Model file for the job. Use its own axes, mm. A direction names the side the tool comes from. Round coordinates to 2 decimals unless told otherwise and drop trailing zeros. Order: outer loops, then holes, each group sorted by start corner. A loop starts at its lowest first (then second) coordinate and runs counter-clockwise, first axis right, second up. Notation, with made-up numbers: (29, 45.25) - (58, 45.25) arc R26 cw to (58, 61.25) - close; hole circle Ø4 at (24, 35). An arc over 180 degrees is marked (long way). Put each result on its own line as item: value. Start each with the question number.
Item 1: Mould opens along Z. For faces 4 (the face through (2, 13, 2.075)), 5 (the face through (-1.5, 5.42, 0.07)), 6 (the face through (3, 15, -2.095)) say: pulls with the +Z half, pulls with the -Z half, needs draft (parallel to the pull), parting line crosses it, or undercut.
Item 2: Pin check, flat tips, straight feed: pin 1 Ø0.9 at (x, z) = (0, 0.5) entering from -Y; pin 2 Ø2 at (x, y) = (-2.5, 4) entering from -Z; pin 3 Ø3 at (x, y) = (2.5, 13.5) entering from +Z (3 decimals). Stop position of each tip, or through.
Item 3: Saw through at B-B on z = 0. List the corners of the cut face in (x, y).
Item 4: Saw through at D-D on z = -1.85. List the corners of the cut face in (x, y), plus the area to 3 significant figures.
Item 5: Saw through at C-C on y = 3.25. List the corners of the cut face in (x, z), plus the area to 3 significant figures.
Item 6: Which spindle directions (+Z, -Z, +X, -X, +Y, -Y) get a long thin tool onto all of the face, cutting with end or side? Do faces 1 (the face through (1.2, 12, -2.075)), 2 (the face through (-0.029, 10.166, 2.409)), 3 (the face through (-2.947, 5.916, -0.13)). Say none if no direction does.
Item 7: Probe probe 1 along Z at (x, y) = (0, 7.5); probe 2 along Z at (x, y) = (2.5, 16.75) (3 decimals); probe 3 along X at (y, z) = (13.25, -1.8). List the from-to ranges inside material, lowest first.
Item 8: Saw through at A-A on x = 0. List the corners of the cut face in (y, z) (3 decimals), plus the area to 3 significant figures.
```python
from build123d import *

# Parameters (mm, degrees)
SKETCH1_R               = 2.95
BOSS_EXTRUDE1_DEPTH     = 12
SKETCH5_R               = 1.5
CUT_EXTRUDE3_DEPTH      = 11
CUT_EXTRUDE4_DEPTH      = 5.5
CUT_EXTRUDE4_DEPTH_BACK = 5.5
SKETCH12_R              = 3.400000058
SKETCH12_R_2            = 2.501374622
BOSS_EXTRUDE5_DEPTH     = 0.02


with BuildPart() as part:
    # Sketch1 → Boss-Extrude1 (new body)
    with BuildSketch(Plane(origin=(0, 0, 0), x_dir=(1, 0, 0), z_dir=(0, 1, 0))):
        Circle(SKETCH1_R)
    extrude(amount=BOSS_EXTRUDE1_DEPTH)

    # Sketch5 → Cut-Extrude3 (cut)
    with BuildSketch(Plane.XZ):
        Circle(SKETCH5_R)
    extrude(amount=-CUT_EXTRUDE3_DEPTH, mode=Mode.SUBTRACT)

    # Sketch2 → Revolve3 (revolve)
    with BuildSketch(Plane(origin=(0, 0, 0), x_dir=(0, 0, -1), z_dir=(1, 0, 0))):
        with BuildLine():
            Line((0, 19.898161268), (0, 10.898161268))
            ThreePointArc((0, 10.898161268), (4.5, 15.398161268), (0, 19.898161268))
        make_face()
    revolve(axis=Axis((0, 12, 0), (0, -1, 0)))

    # Sketch8 → Cut-Extrude4 (cut, two sides)
    with BuildSketch(Plane(origin=(0, 0, 0), x_dir=(0, 0, -1), z_dir=(1, 0, 0))) as cut_extrude4_sk:
        Polygon((-2.075, 20.390789919), (-2.075, 10.5), (-5.08, 7.495), (-5.08, 20.390789919), align=None)
        Polygon((5.08, 20.390789919), (2.075, 20.390789919), (2.075, 10.5), (5.08, 7.495), align=None)
    extrude(amount=CUT_EXTRUDE4_DEPTH, mode=Mode.SUBTRACT)
    extrude(cut_extrude4_sk.sketch, amount=-CUT_EXTRUDE4_DEPTH_BACK, mode=Mode.SUBTRACT)

    # Sketch11 → Cut-Revolve2 (revolve, cut)
    with BuildSketch(Plane(origin=(0, 0, 0), x_dir=(0, 0, -1), z_dir=(1, 0, 0))):
        with BuildLine():
            Line((-3.25, 15.398161268), (3.25, 15.398161268))
            ThreePointArc((3.25, 15.398161268), (0, 18.648161268), (-3.25, 15.398161268))
        make_face()
    revolve(axis=Axis((0, 15.398161268, 2.075), (0, 0, -1)), mode=Mode.SUBTRACT)

    # Sketch12 → Boss-Extrude5 (add)
    with BuildSketch(Plane(origin=(0, 0, -2.075), x_dir=(-1, 0, 0), z_dir=(0, 0, -1))):
        with Locations((0, 15.398161268)):
            Circle(SKETCH12_R)
        with Locations((0, 15.398161268)):
            Circle(SKETCH12_R_2, mode=Mode.SUBTRACT)
    extrude(amount=BOSS_EXTRUDE5_DEPTH)


solid = part.part
```
Results found:
1. face 4: pulls with the +Z half
1. face 5: undercut
1. face 6: pulls with the -Z half
2. pin 1: stops at y = 10.9
2. pin 2: stops at z = -2.54
2. pin 3: stops at z = 2.075
3. outline: (-2.95, 0) - (-1.5, 0) - (-1.5, 11) - (-0.95, 11) arc R4.5 ccw to (0.95, 11) - (1.5, 11) - (1.5, 0) - (2.95, 0) - (2.95, 12) arc R4.5 ccw (long way) to (-2.95, 12) - close; hole circle Ø6.5 at (0, 15.4)
4. outline: (-2.3, 0) - (2.3, 0) - (2.3, 12) arc R4.1 ccw (long way) to (-2.3, 12) - close; hole circle Ø5.34 at (0, 15.4)
4. area: 83.4 mm²
5. outline: circle Ø5.9 at (0, 0); hole circle Ø3 at (0, 0)
5. area: 20.3 mm²
6. face 1: -Z
6. face 2: +Z, +X, -X, +Y
6. face 3: -Y
7. probe 1: z = -2.95 to -1.5, 1.5 to 2.95
7. probe 2: z = -2.095 to -1.576, 1.576 to 2.075
7. probe 3: x = -3.52 to -1.65, 1.65 to 3.52
8. outline: (0, -2.95) - (9.625, -2.95) - (10.5, -2.075) - (11.998, -2.075) - (11.998, -2.095) - (12.897, -2.095) - (12.897, -2.075) arc R3.25 cw to (12.897, 2.075) - (10.5, 2.075) - (9.625, 2.95) - (0, 2.95) - (0, 1.5) - (11, 1.5) - (11, 0.952) arc R4.5 ccw to (11, -0.952) - (11, -1.5) - (0, -1.5) - close; (17.9, -2.095) - (18.798, -2.095) - (18.798, -2.075) - (19.391, -2.075) arc R4.5 ccw to (19.391, 2.075) - (17.9, 2.075) arc R3.25 cw to (17.9, -2.075) - close
8. area: 41.7 mm²
